Geometry: final body of the model. Coordinates: model frame, mm. A direction names the side the tool comes from. Round coordinates to 2 decimals unless told otherwise and drop trailing zeros. Loops run counter-clockwise (first coordinate to the right, second up) from the corner with the lowest first, then second, coordinate; pieces in that order, holes last. Notation, with made-up numbers: (47, 37.25) -> (56, 37.25) arc R18 ccw to (56, 63.25) -> close; hole circle Ø3 at (-4.75, -0.5). An arc over 180 degrees is marked (long way). Answer in a Markdown table with one row per item.
Autodesk Inventor part; units mm, degrees
ref_plane "YZ Plane" through (0, 0, 0) normal (1, 0, 0) x (0, 1, 0)
ref_plane "XZ Plane" through (0, 0, 0) normal (0, 1, 0) x (-1, 0, 0)
ref_plane "XY Plane" through (0, 0, 0) normal (0, 0, 1) x (1, 0, 0)
sketch "スケッチ1" plane through (0, 0, 0) normal (0, 0, 1) x (1, 0, 0)
  line L0 (-59.5, -21.75) -> (59.5, -21.75) construction
  line L1 (59.5, -21.75) -> (59.5, 21.75) construction
  line L2 (59.5, 21.75) -> (-59.5, 21.75) construction
  line L3 (-59.5, 21.75) -> (-59.5, -21.75) construction
  line L4 (-59.5, -21.75) -> (59.5, 21.75) construction
  line L5 (59.5, -21.75) -> (-59.5, 21.75) construction
  line L6 (-54.5, -16.75) -> (54.5, -16.75) construction
  line L7 (54.5, -16.75) -> (54.5, 16.75) construction
  line L8 (54.5, 16.75) -> (-54.5, 16.75) construction
  line L9 (-54.5, 16.75) -> (-54.5, -16.75) construction
  line L10 (-54.5, -16.75) -> (54.5, 16.75) construction
  line L11 (54.5, -16.75) -> (-54.5, 16.75) construction
  line L12 (-33.05, 11.05) -> (-27.95, 11.05)
  line L13 (-27.95, 11.05) -> (-27.95, -4.05)
  line L14 (-27.95, -4.05) -> (-33.05, -4.05)
  line L15 (-33.05, -4.05) -> (-33.05, 11.05)
  line L16 (-28, 11) -> (-33, 11) construction
  line L17 (-33, 11) -> (-33, -4) construction
  line L18 (-33, -4) -> (-28, -4) construction
  line L19 (-28, -4) -> (-28, 11) construction
  line L20 (-30.5, 11) -> (-30.5, -4) construction
  line L21 (-33, 21) -> (-28, 21) construction
  line L22 (-28, 21) -> (-28, -14) construction
  line L23 (-28, -14) -> (-33, -14) construction
  line L24 (-33, -14) -> (-33, 21) construction
  circle A0 centre (-30.5, 17) radius 1.55
  circle A1 centre (-30.5, -10) radius 1.55
  circle A2 centre (-33.05, 10) radius 1.05
  circle A3 centre (-27.95, 10) radius 1.05
  circle A4 centre (-33.05, -3) radius 1.05
  circle A5 centre (-27.95, -3) radius 1.05
  line L25 (0, 0) -> (0, 16.75) construction
  line L26 (0, 0) -> (54.5, 0) construction
  circle A6 centre (30.5, 17) radius 1.55
  circle A7 centre (30.5, -10) radius 1.55
  circle A8 centre (27.95, 10) radius 1.05
  circle A9 centre (33.05, 10) radius 1.05
  circle A10 centre (27.95, -3) radius 1.05
  circle A11 centre (33.05, -3) radius 1.05
  line L27 (33.05, 11.05) -> (27.95, 11.05)
  line L28 (27.95, 11.05) -> (27.95, -4.05)
  line L29 (27.95, -4.05) -> (33.05, -4.05)
  line L30 (33.05, -4.05) -> (33.05, 11.05)
  line L31 (-59.5, 11.75) -> (-62.5, 11.75)
  line L32 (-62.5, 11.75) -> (-62.5, -11.75)
  line L33 (-62.5, -11.75) -> (-59.5, -11.75)
  line L34 (-59.5, 13.85) -> (-59.5, 21.75)
  line L35 (-59.5, 21.75) -> (-21.6, 21.75)
  line L36 (-19.5, 21.75) -> (-19.5, 26.75)
  line L37 (-19.5, 26.75) -> (19.5, 26.75)
  line L38 (19.5, 26.75) -> (19.5, 21.75)
  line L39 (21.6, 21.75) -> (59.5, 21.75)
  line L40 (59.5, 21.75) -> (59.5, 13.85)
  line L41 (59.5, 11.75) -> (62.5, 11.75)
  line L42 (62.5, 11.75) -> (62.5, -11.75)
  line L43 (62.5, -11.75) -> (59.5, -11.75)
  line L44 (-59.5, -13.85) -> (-59.5, -21.75)
  line L45 (-59.5, -21.75) -> (59.5, -21.75)
  line L46 (59.5, -21.75) -> (59.5, -13.85)
  arc A12 (-59.5, 11.75) -> (-59.5, 13.85) centre (-59.5, 12.8) ccw
  arc A13 (-59.5, -13.85) -> (-59.5, -11.75) centre (-59.5, -12.8) ccw
  line L47 (0, 0) -> (-54.5, 0) construction
  arc A14 (59.5, -11.75) -> (59.5, -13.85) centre (59.5, -12.8) ccw
  arc A15 (59.5, 13.85) -> (59.5, 11.75) centre (59.5, 12.8) ccw
  arc A16 (-21.6, 21.75) -> (-19.5, 21.75) centre (-20.55, 21.75) ccw
  arc A17 (19.5, 21.75) -> (21.6, 21.75) centre (20.55, 21.75) ccw
  line L48 (-56.8855, 19.3) -> (-54.5, 19.3) construction
  line L49 (-54.5, 19.3) -> (-54.5, 16.2) construction
  line L50 (-54.5, 16.2) -> (-56.8855, 16.2) construction
  line L51 (-56.8855, 16.2) -> (-56.8855, 19.3) construction
  line L52 (-54.5, 17.75) -> (-56.8855, 17.75) construction
  line L53 (-53.05, 22.7202) -> (-49.95, 22.7202) construction
  line L54 (-49.95, 22.7202) -> (-49.95, 16.75) construction
  line L55 (-49.95, 16.75) -> (-53.05, 16.75) construction
  line L56 (-53.05, 16.75) -> (-53.05, 22.7202) construction
  line L57 (-51.5, 22.7202) -> (-51.5, 16.75) construction
  point P0 (-30.5, -14)
  dimension "d10" = 2.1
  dimension "d0" = 33.5
  dimension "d1" = 5
  dimension "d2" = 109
  dimension "d3" = 5
  dimension "d4" = 0.05
  dimension "d5" = 35
  dimension "d6" = 27
  dimension "d7" = 5
  dimension "d11" = 33
  dimension "d12" = 3.1
  dimension "d13" = 1.05
  dimension "d14" = 3
  dimension "d15" = 4
  dimension "d16" = 3.1
  dimension "d17" = 10
  dimension "d18" = 5
  dimension "d19" = 8
  dimension "d20" = 5
  dimension "d21" = 40
  dimension "d22" = 5
  dimension "d50" = 4
  dimension "d51" = 10
  dimension "d52" = 17
  dimension "d53" = 10
extrude "押し出し1" add sketch "スケッチ1" along normal blind 5
ref_plane "作業平面1" through (23, -13.75, 5) normal (-1, 0, 0) x (0, 0, 1)
sketch "スケッチ7" plane through (23, -13.75, 5) normal (-1, 0, 0) x (0, 0, 1)
  point P0 (-5, 13.75)
sketch "スケッチ9" plane through (0, 0, 5) normal (0, 0, 1) x (1, 0, 0)
  circle A0 centre (-30.5, 17) radius 1.55
  circle A1 centre (-30.5, 17) radius 1.55
  circle A2 centre (-30.5, -10) radius 1.55
  circle A3 centre (-30.5, -10) radius 1.55
  circle A4 centre (30.5, 17) radius 1.55
  circle A5 centre (30.5, 17) radius 1.55
  circle A6 centre (30.5, -10) radius 1.55
  circle A7 centre (30.5, -10) radius 1.55
  point P0 (0, 0)
extrude "押し出し5" add sketch "スケッチ9" against normal up to surface (5 mm away)
equation "\"d20\" = d18"
equation "\"d53\" = d51"
properties part number "コックピット_サブフレーム_1_3" material "アセタール樹脂、黒"
Item 1: Cut plane A-A (x = -49). Output: boundary loops of the cut face in (y, z), then the cut area to 4 significant figures.
Answer:
| item | result |
|---|---|
| outline | (-21.75, 0) -> (21.75, 0) -> (21.75, 5) -> (-21.75, 5) -> close |
| area | 217.5 mm² |
Item 2: Reachability of faces 1 (the face through (-61, -11.75, 2)), 2 (the face through (-41, 21.75, 2)), 3 (the face through (31, 11.05, 2)), 4 (the face through (62.5, 0, 2)), 5 (the face through (59.5, 18, 2)) from +Z, -Z, +X, -X, +Y, -Y: full face, straight path, thin tool, end or side. Return the list, or none.
Answer:
| item | result |
|---|---|
| face 1 | +Z, -Z, -X, -Y |
| face 2 | +Z, -Z, -X, +Y |
| face 3 | +Z, -Z |
| face 4 | +Z, -Z, +X, +Y, -Y |
| face 5 | +Z, -Z, +X, +Y |
Item 3: Line query: probe 1 along X at (y, z) = (21.5, 1.4); probe 2 along X at (y, z) = (4, 3.5); probe 3 along Y at (x, z) = (29, 0.7). Output: solid intervals per line, ascending. Write a range as [from, to].
Answer:
| item | result |
|---|---|
| probe 1 | x = [-59.5, -21.57], [-19.53, 19.53], [21.57, 59.5] |
| probe 2 | x = [-62.5, -33.05], [-27.95, 27.95], [33.05, 62.5] |
| probe 3 | y = [-21.75, -4.05], [11.05, 21.75] |
Item 4: Cut plane B-B (z = 3.9). Count the separate pieces of the cut face and the enclosed holes in it, then the cut area to 3 significant figures.
Answer:
| item | result |
|---|---|
| separate pieces | 1 |
| enclosed holes | 2 |
| area | 5,330 mm² |
Item 5: Draft query along Y for faces 6 (the face through (26.9, 10, 2.5)), 7 (the face through (19.5, 24, 2)), 8 (the face through (-1, -21.75, 2)). Return one class per face: pulls with the +Y half, pulls with the -Y half, needs draft (parallel to the pull), parting line crosses it, or undercut.
Answer:
| item | result |
|---|---|
| face 6 | undercut |
| face 7 | needs draft |
| face 8 | pulls with the -Y half |
Item 6: Pin query (flat end, axial travel): pin 1 Ø2.5 at (x, z) = (-47, 2) entering from +Y; pin 2 Ø2.5 at (x, z) = (-61.5, 2) entering from -Y; pin 3 Ø8 at (x, y) = (37.5, 11) entering from -Z; pin 4 Ø1.5 at (x, z) = (-61, 2.5) entering from +Y. Return the tip coordinate at first contact, or that it passes through.
Answer:
| item | result |
|---|---|
| pin 1 | stops at y = 21.75 |
| pin 2 | stops at y = -11.75 |
| pin 3 | stops at z = 0 |
| pin 4 | stops at y = 11.75 |
